Geometry check sheet. Reference: the model listing, model coordinates, mm. A direction names the side the tool comes from. Give positions to 0.01 mm unless a question says otherwise; leave off trailing zeros. Loops run counter-clockwise (first coordinate to the right, second up) from the corner with the lowest first, then second, coordinate; pieces in that order, holes last. Notation, with made-up numbers: (-31.5, 86.5) -> (16.5, 86.5) arc R29 cw to (16.5, 120.5) -> close; hole circle Ø7 at (-27.75, 37.25). An arc over 180 degrees is marked (long way). Answer in a Markdown table with one row per item. Add a question column.
```python
from build123d import *

# Parameters (mm, degrees)
F1_DEPTH = 25.4
F3_DEPTH = 76.2


with BuildPart() as f1:
    # F0 (on Top) → F1 (new body)
    with BuildSketch(Plane.XY):
        Polygon((-35.135657, 0), (-9.735657, 0), (-9.735657, 127), (-35.135657, 127), (-35.135657, 101.6), (-25.610657, 101.6), (-25.610657, 76.2), (-35.135657, 76.2), align=None)
    extrude(amount=F1_DEPTH)

    # F2 (on face) → F3 (join)
    with BuildSketch(Plane.XY.offset(25.4)):
        Polygon((-35.135657, 76.2), (-35.135657, 0), (-9.735657, 0), (-9.735657, 127), (-35.135657, 127), (-35.135657, 101.6), (-25.610657, 101.6), (-25.610657, 76.2), align=None)
    extrude(amount=F3_DEPTH)


solid = f1.part
```
1. Sectioned sample at B-B (z = 8.5). Enter the section's corners in (x, y), plus the area to 3 significant figures.
2. Release check for a two-part mould opening along Y. For faces 1 (the face through (-22, 127, 50)), 2 (the face through (-30, 101.6, 50)), 3 (the face through (-25.611, 89, 50)), 4 (the face through (-35.136, 39, 50)) record: released by +Y, released by -Y, zero draft, split by the parting line, or undercut.
3. Sectioned sample at C-C (y = 80.5). Enter the section's corners in (x, z).
4. Access from +Z, -Z, +X, -X, +Y, -Y to the whole of each face (thin tool, end or side, straight path). Record for faces 5 (the face through (-23, 64, 0)), 6 (the face through (-30, 76.2, 50)).
5. Gauge pin test, flat end, axial feed: pin 1 Ø7.5 at (y, z) = (91, 73.5) entering from -X. Record the tip position at first contact, or that the pin passes through.
6. Sectioned sample at A-A (x = -31.5). Enter the section's corners in (y, z).
7. Material ranges on L1, parallel to Y at x = -30.5, z = 73.5; L2, parallel to X at y = 97.5, z = 81.5, recorded low to high. Write a range as from..to.
Response:
| question | item | result |
|---|---|---|
| 1 | outline | (-35.14, 0) -> (-9.74, 0) -> (-9.74, 127) -> (-35.14, 127) -> (-35.14, 101.6) -> (-25.61, 101.6) -> (-25.61, 76.2) -> (-35.14, 76.2) -> close |
| 1 | area | 2,980 mm2 |
| 2 | face 1 | released by +Y |
| 2 | face 2 | undercut |
| 2 | face 3 | undercut |
| 2 | face 4 | zero draft |
| 3 | outline | (-25.61, 0) -> (-9.74, 0) -> (-9.74, 101.6) -> (-25.61, 101.6) -> close |
| 4 | face 5 | -Z, +X, -X, +Y, -Y |
| 4 | face 6 | +Z, -Z, -X |
| 5 | pin 1 | stops at x = -25.61 |
| 6 | outline | (0, 0) -> (76.2, 0) -> (76.2, 101.6) -> (0, 101.6) -> close; (101.6, 0) -> (127, 0) -> (127, 101.6) -> (101.6, 101.6) -> close |
| 7 | L1 | y = 0..76.2, 101.6..127 |
| 7 | L2 | x = -25.61..-9.74 |
